The listing builds one solid part. Answer for the finished solid, in the listing's coordinates (mm). Round coordinates to 2 decimals unless told otherwise and drop trailing zeros. Write each loop counter-clockwise with the first axis right and the second up, starting at its lowest first coordinate (ties: lowest second). Pieces come first, ordered by that corner, then holes. Notation, with made-up numbers: M 47.25,-0.5 L 86.25,-0.5 A31 ccw 86.25,33.5 Z; hole C -14.75,78 d2. An arc over 180 degrees is marked long. One line per item, written item: value. Start each with the question number.
(1) Consider probe 1 along X at (y, z) = (0.5, 0); probe 2 along Z at (x, y) = (4, 0.85); probe 3 along X at (y, z) = (-0.75, 10). Determine where each line is inside the solid, lowest interval first.
(2) Section B-B (y = 0.35) is taken. Determine the outline of the cut face in (x, z).
(3) Section C-C (x = 3.5) is taken. Determine the outline of the cut face in (y, z).
(4) Section A-A (z = 9) is taken. Determine the outline of the cut face in (x, y), plus the area to 3 significant figures.
(5) Section D-D (z = -4.5) is taken. Determine the outline of the cut face in (x, y), plus the area to 3 significant figures.
(6) Given P1, Ø1, axis at x = 3.5, y = 0, coming from the +Z side; P2, Ø0.5, axis at x = 5, y = 0.5, coming from the -Z side; P3, Ø1, axis at y = 0.5, z = 9, coming from the -X side, each flat-ended and moving along its own axis, determine where each tip first touches the part or whether it passes through.
```python
from build123d import *

# Parameters (mm, degrees)
PAD_DEPTH = 1


with BuildPart() as part:
    # Sketch → Pad (new body, symmetric)
    with BuildSketch(Plane.XZ):
        with BuildLine():
            Line((-15, -12), (4.5, -12))
            Line((4.5, -10.45), (4.5, -12))
            Line((6.2, -10.45), (4.5, -10.45))
            Line((6.2, -12), (6.2, -10.45))
            Line((6.2, -12), (9, -12))
            Line((9, -12), (9, 12))
            Line((9, 12), (5.3, 12))
            Line((5.3, 7), (5.3, 12))
            Line((1.5, 7), (5.3, 7))
            Line((1.5, 12), (1.5, 7))
            Line((1.5, 12), (-15, 12))
            ThreePointArc((-15, 12), (-27, 0), (-15, -12))
        make_face()
    extrude(amount=PAD_DEPTH, both=True)


solid = part.part
```
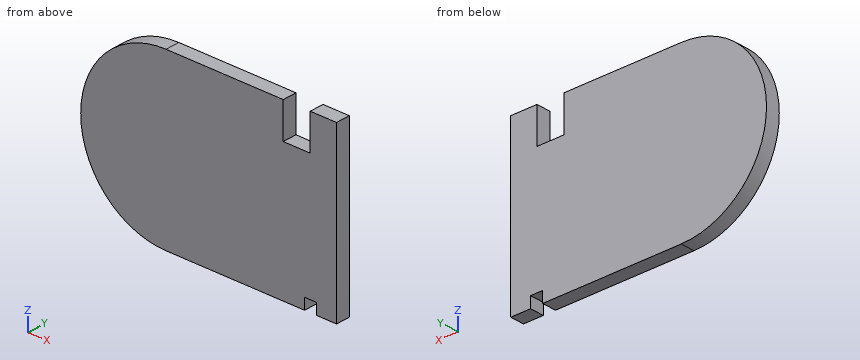
Recorded:
1. probe 1: x = -27 to 9
1. probe 2: z = -12 to 7
1. probe 3: x = -21.63 to 1.5, 5.3 to 9
2. outline: M -15,-12 L 4.5,-12 L 4.5,-10.45 L 6.2,-10.45 L 6.2,-12 L 9,-12 L 9,12 L 5.3,12 L 5.3,7 L 1.5,7 L 1.5,12 L -15,12 A12 ccw Z
3. outline: M -1,-12 L 1,-12 L 1,7 L -1,7 Z
4. outline: M -22.94,-1 L 1.5,-1 L 1.5,1 L -22.94,1 Z; M 5.3,-1 L 9,-1 L 9,1 L 5.3,1 Z
4. area: 56.3 mm2
5. outline: M -26.12,-1 L 9,-1 L 9,1 L -26.12,1 Z
5. area: 70.2 mm2
6. P1: stops at z = 7
6. P2: stops at z = -10.45
6. P3: stops at x = -23.47
